Can you work these out from the model? Positions are in its coordinate system, mm. Give positions to 0.01 mm unless a question says otherwise; leave off trailing zeros. Order: outer loops, then holes, each group sorted by start corner. A loop starts at its lowest first (then second) coordinate and runs counter-clockwise, first axis right, second up. Notation, with made-up numbers: (55.5, 7.5) - (61.5, 7.5) arc R20 ccw to (61.5, 12.5) - close; hole circle Ø10 at (72.5, 4). An arc over 180 degrees is marked (long way). Return JSON: item names as keys, results as strings.
```python
from build123d import *

# Parameters (mm, degrees)
SKETCH_W        = 150
SKETCH_H        = 120
PAD_DEPTH       = 3
SKETCH002_W     = 120
SKETCH002_H     = 90
POCKET_DEPTH    = 5
SKETCH001_W     = 140
SKETCH001_H     = 100
POCKET001_DEPTH = 1.5
SKETCH003_R     = 2
POCKET002_DEPTH = 5
SKETCH004_R     = 2
POCKET003_DEPTH = 5
SKETCH005_R     = 2
POCKET004_DEPTH = 5
SKETCH006_R     = 2
POCKET005_DEPTH = 5
FILLET_R        = 1.9


with BuildPart() as part:
    # Sketch → Pad (new body)
    with BuildSketch(Plane.XY):
        with Locations((75, 60)):
            Rectangle(SKETCH_W, SKETCH_H)
    extrude(amount=-PAD_DEPTH)

    # Sketch002 → Pocket (cut)
    with BuildSketch(Plane.XY):
        with Locations((75, 60)):
            Rectangle(SKETCH002_W, SKETCH002_H)
    extrude(amount=-POCKET_DEPTH, mode=Mode.SUBTRACT)

    # Sketch001 → Pocket001 (cut)
    with BuildSketch(Plane.XY):
        with Locations((75, 60)):
            Rectangle(SKETCH001_W, SKETCH001_H)
    extrude(amount=-POCKET001_DEPTH, mode=Mode.SUBTRACT)

    # Sketch003 → Pocket002 (cut)
    with BuildSketch(Plane.XY):
        with Locations((10, 20)):
            Circle(SKETCH003_R)
    extrude(amount=-POCKET002_DEPTH, mode=Mode.SUBTRACT)

    # Sketch004 → Pocket003 (cut)
    with BuildSketch(Plane.XY):
        with Locations((10, 100)):
            Circle(SKETCH004_R)
    extrude(amount=-POCKET003_DEPTH, mode=Mode.SUBTRACT)

    # Sketch005 → Pocket004 (cut)
    with BuildSketch(Plane.XY):
        with Locations((140, 20)):
            Circle(SKETCH005_R)
    extrude(amount=-POCKET004_DEPTH, mode=Mode.SUBTRACT)

    # Sketch006 → Pocket005 (cut)
    with BuildSketch(Plane.XY):
        with Locations((140, 100)):
            Circle(SKETCH006_R)
    extrude(amount=-POCKET005_DEPTH, mode=Mode.SUBTRACT)

    # Fillet
    fillet_edges = [part.edges().sort_by_distance(p)[0] for p in [
        (0, 60, 0),
        (75, 0, 0),
        (150, 60, 0),
        (75, 120, 0),
        (0, 0, -1.5),
        (150, 0, -1.5),
        (150, 120, -1.5),
        (0, 120, -1.5),
    ]]
    fillet(fillet_edges, radius=FILLET_R)


solid = part.part
```
1. If I drill on L1, parallel to Y at x = 10, z = -2.7; L2, parallel to X at y = 71, z = -1.8; L3, parallel to Y at x = 100, z = -2.05, over which ranges is the centre line in solid material (lowest first)? Write a range as [from, to].
Checks:
{"L1": "[0, 18], [22, 98], [102, 120]", "L2": "[0, 15], [135, 150]", "L3": "[0, 15], [105, 120]"}
2. Suppose I cut it at A-A (y = 87.5). List the corners of the cut face in (x, z) for me.
Checks:
{"outline": "(0, -3) - (15, -3) - (15, -1.5) - (5, -1.5) - (5, 0) - (1.9, 0) arc R1.9 ccw to (0, -1.9) - close; (135, -3) - (150, -3) - (150, -1.9) arc R1.9 ccw to (148.1, 0) - (145, 0) - (145, -1.5) - (135, -1.5) - close"}
3. Suppose I cut it at C-C (y = 20). List the corners of the cut face in (x, z) for me.
Checks:
{"outline": "(0, -3) - (8, -3) - (8, -1.5) - (5, -1.5) - (5, 0) - (1.9, 0) arc R1.9 ccw to (0, -1.9) - close; (12, -3) - (15, -3) - (15, -1.5) - (12, -1.5) - close; (135, -3) - (138, -3) - (138, -1.5) - (135, -1.5) - close; (142, -3) - (150, -3) - (150, -1.9) arc R1.9 ccw to (148.1, 0) - (145, 0) - (145, -1.5) - (142, -1.5) - close"}
4. Thinking about a two-plate mould opening in Y: for faces 1 (the face through (74, 114, -3)), 2 (the face through (75, 108, -1.5)), which applies, +Y half, -Y half, draft (parallel to the pull), parting line (faces both ways), or undercut?
Checks:
{"face 1": "draft", "face 2": "undercut"}
5. For pin 1 Ø1.6 at (y, z) = (83, -0.5) entering from -X; pin 2 Ø3.5 at (x, y) = (10, 20) entering from +Z; pin 3 Ø4.5 at (x, y) = (140, 20) entering from +Z; pin 4 Ø0.8 at (x, z) = (57, -0.5) entering from +Y, each with a flat end and sliding along its axis, tell me the tip position at first contact or that it passes through.
Checks:
{"pin 1": "x = 0.1", "pin 2": "through", "pin 3": "z = -1.5", "pin 4": "y = 119.72"}
6. Suppose I cut it at B-B (x = 21). List the corners of the cut face in (y, z) for me, plus the area to 3 significant figures.
Checks:
{"outline": "(0, -3) - (15, -3) - (15, -1.5) - (10, -1.5) - (10, 0) - (1.9, 0) arc R1.9 ccw to (0, -1.9) - close; (105, -3) - (120, -3) - (120, -1.9) arc R1.9 ccw to (118.1, 0) - (110, 0) - (110, -1.5) - (105, -1.5) - close", "area": "73.5 mm^2"}
7. Suppose I cut it at D-D (z = -2.55). List the corners of the cut face in (x, y) for me.
Checks:
{"outline": "(0, 1.9) arc R1.9 ccw to (1.9, 0) - (148.1, 0) arc R1.9 ccw to (150, 1.9) - (150, 118.1) arc R1.9 ccw to (148.1, 120) - (1.9, 120) arc R1.9 ccw to (0, 118.1) - close; hole circle Ø4 at (10, 20); hole circle Ø4 at (10, 100); hole (15, 15) - (135, 15) - (135, 105) - (15, 105) - close; hole circle Ø4 at (140, 20); hole circle Ø4 at (140, 100)"}
